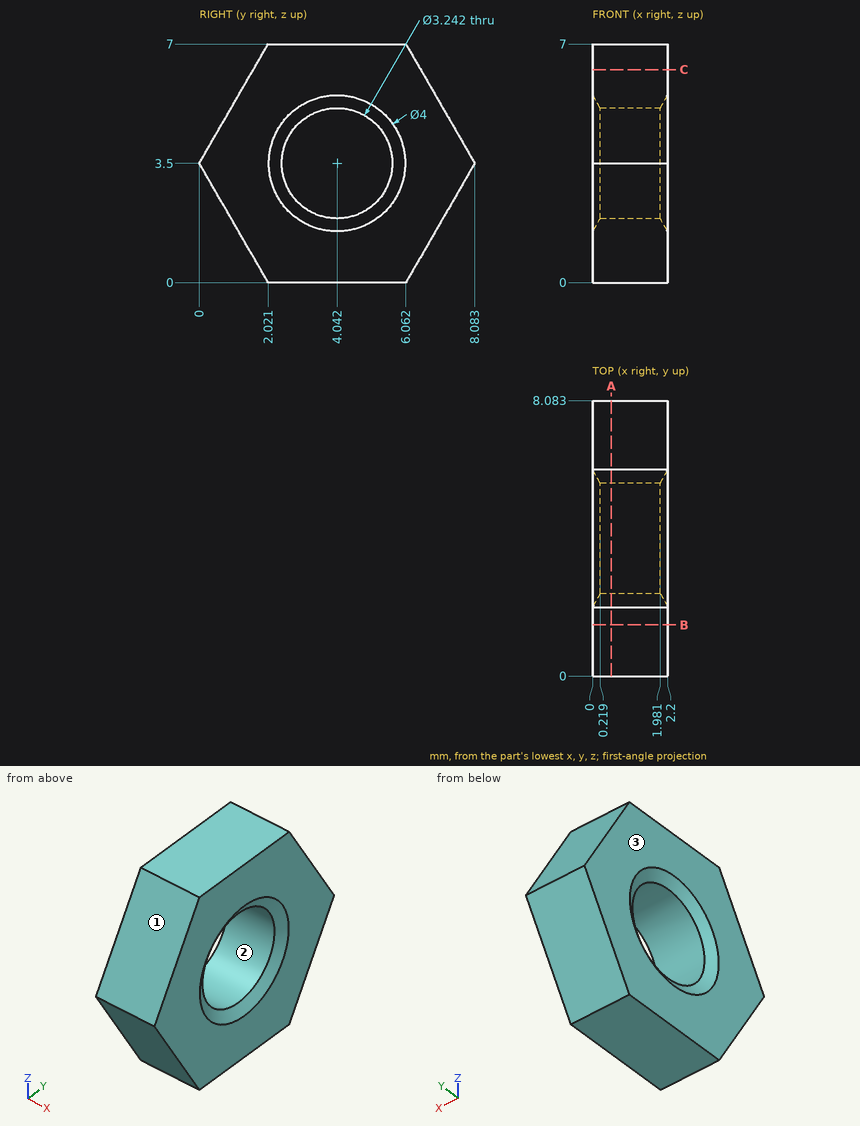
Job drawing, mm, ordinate dimensions from the low corner. One solid piece. Give positions to 0.01 mm unless a question says otherwise; leave off trailing zeros. Write each loop counter-clockwise with the first axis right and the second up, starting at its lowest first coordinate (ties: lowest second). Pieces come first, ordered by that corner, then holes. Notation, with made-up numbers: (43.5, -27) - (72.5, -27) arc R35 cw to (72.5, 7) - close; hole circle Ø3 at (68, 14). An arc over 180 degrees is marked (long way). Use one line per item in the form item = value. Start each with the question number.
1. Band-saw the part on B-B on y = 1.5. Write the cut outline in (x, z), plus the area to 3 significant figures.
2. Band-saw the part on C-C on z = 6.25. Write the cut outline in (x, y) (1 decimal), plus the area to 3 significant figures.
3. Probe line 1 (Z direction, x = 0.3, y = 4); line 2 (Y direction, x = 1.1, z = 4.5) (1 decimal); line 3 (Y direction, x = 0.5, z = 6.75) (1 decimal). List the from-to ranges inside material, lowest first. Write a range as [from, to].
4. Band-saw the part on A-A on x = 0.55. Write the cut outline in (y, z).
5. Two-plate mould, pull along Z, no slides. Class the marked faces 1, 2 and 3: released by +Z, released by -Z, zero draft, split by the parting line, or undercut.
6. Drop a flat-ended pin along its axis: pin 1 Ø3.5 at (y, z) = (4.04, 3.5) entering from +X. Give the stop position or say it passes through.
Conclusion:
q1.outline = (0, 0.9) - (2.2, 0.9) - (2.2, 6.1) - (0, 6.1) - close
q1.area = 11.4 mm²
q2.outline = (0, 1.6) - (2.2, 1.6) - (2.2, 6.5) - (0, 6.5) - close
q2.area = 10.8 mm²
q3.line_1 = [0, 1.88], [5.12, 7]
q3.line_2 = [0.6, 2.8], [5.3, 7.5]
q3.line_3 = [1.9, 6.2]
q4.outline = (0, 3.5) - (2.02, 0) - (6.06, 0) - (8.08, 3.5) - (6.06, 7) - (2.02, 7) - close; hole circle Ø3.24 at (4.04, 3.5)
q5.face_1 = released by +Z
q5.face_2 = undercut
q5.face_3 = zero draft
q6.pin_1 = 2.06
